```python
from build123d import *

# Parameters (mm, degrees)
F1_DEPTH = 31.75
F3_R     = 1.27
F4_R     = 4.7625
F4_R_2   = 4.1275
F5_DEPTH = 3.175
F6_R     = 4.7625
F6_R_2   = 4.1275
F7_DEPTH = 3.175


# Not quite as in the source:
# - a feature of the source that left no trace in its solid (it failed there, or was rolled back) is left out


with BuildPart() as f1:
    # F0 (on Right) → F1 (new body)
    with BuildSketch(Plane.YZ):
        Polygon((0, 203.2), (-304.8, 203.2), (-304.8, 200.025), (-228.6, 200.025), (-3.175, 76.2), (-3.175, 0), (0, 0), align=None)
        Polygon((-222.0052667175, 200.025), (-3.175, 200.025), (-3.175, 79.822459127), align=None, mode=Mode.SUBTRACT)
    extrude(amount=F1_DEPTH)

    # F3
    f3_edges = [f1.edges().sort_by_distance(p)[0] for p in [
        (15.875, -3.175, 79.822459),
        (15.875, -222.005267, 200.025),
        (15.875, -3.175, 200.025),
        (15.875, 0, 203.2),
        (15.875, -304.8, 203.2),
        (0, -152.4, 203.2),
        (31.75, -152.4, 203.2),
        (15.875, -304.8, 200.025),
        (0, -304.8, 201.6125),
        (31.75, -304.8, 201.6125),
        (0, -112.590133, 200.025),
        (31.75, -112.590133, 200.025),
        (15.875, 0, 0),
        (0, 0, 101.6),
        (31.75, 0, 101.6),
        (15.875, -3.175, 0),
        (0, -1.5875, 0),
        (31.75, -1.5875, 0),
        (15.875, -228.6, 200.025),
        (0, -266.7, 200.025),
        (31.75, -266.7, 200.025),
        (15.875, -3.175, 76.2),
        (0, -115.8875, 138.1125),
        (31.75, -115.8875, 138.1125),
        (0, -3.175, 38.1),
        (31.75, -3.175, 38.1),
        (0, -112.590133, 139.92373),
        (31.75, -112.590133, 139.92373),
        (0, -3.175, 139.92373),
        (31.75, -3.175, 139.92373),
    ]]
    fillet(f3_edges, radius=F3_R)

    # F4 (on face) → F5 (cut, through all)
    with BuildSketch(Plane(origin=(0, 0, 200.025), x_dir=(1, 0, 0), z_dir=(0, 0, -1))):
        with Locations((15.875, 285.75)):
            Circle(F4_R)
        with Locations((15.875, 247.65)):
            Circle(F4_R)
        with Locations((15.875, 146.05)):
            Circle(F4_R_2)
        with Locations((15.875, 44.45)):
            Circle(F4_R)
    extrude(amount=-F5_DEPTH, mode=Mode.SUBTRACT)

    # F6 (on face) → F7 (cut, through all)
    with BuildSketch(Plane.XZ.offset(3.175)):
        with Locations((15.875, 57.15)):
            Circle(F6_R)
        with Locations((15.875, 19.05)):
            Circle(F6_R)
        with Locations((15.875, 158.75)):
            Circle(F6_R_2)
    extrude(amount=-F7_DEPTH, mode=Mode.SUBTRACT)


solid = f1.part
```
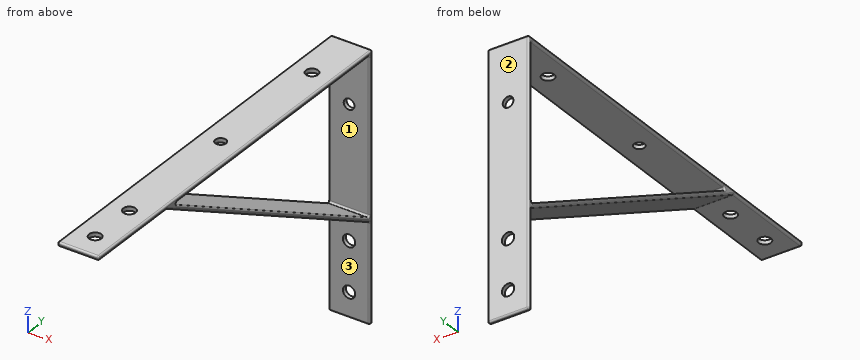
The model under review builds one solid part; all positions refer to its coordinate system, in mm. Face numbers are marked on the shaded views. A direction names the side the tool comes from. Give positions to 0.01 mm unless a question says otherwise; leave off trailing zeros. Write each loop counter-clockwise with the first axis right and the second up, starting at its lowest first coordinate (ties: lowest second). Pieces come first, ordered by that corner, then holes.
(1) Tool access review of the marked faces 1, 2 and 3: name each direction out of +Z, -Z, +X, -X, +Y, -Y from which nothing blocks a thin tool from reaching the whole face with its end or side.
(2) Consider section D-D, the plane z = 158.75. Give the number of separate pieces and of enclosed holes in the cut face, and give its area (3 significant figures).
(3) Consider section C-C, the plane z = 44. Give the boundary of the cut face in (x, y) (3 decimals), and give its area (3 significant figures).
(4) For P1, Ø5.5, axis at x = 15.875, y = -44.45, coming from the +Z side; P2, Ø4, axis at x = 12, y = -41, coming from the -Z side; P3, Ø6.5, axis at x = 15.875, z = 158.75, coming from the +Y side; P4, Ø5.5, axis at x = 15.875, z = 19.05, coming from the +Y side, all flat-tipped, find the tip position at first contact; note any pin that passes through.
(5) To check wall thickness, follow L1, parallel to X at y = -44.45, z = 201.35; L2, parallel to X at y = -44, z = 202; L3, parallel to Z at x = 22, y = -52.5 (3 decimals). State the ranges of each line that lie inside material, in increasing order.
Returned:
1. face 1: +X, -X
1. face 2: +Z, -Z, +X, -X, +Y
1. face 3: -Z, +X, -X, -Y
2. separate pieces: 3
2. enclosed holes: 0
2. area: 280 mm2
3. outline: (0, -1.905) arc R1.27 ccw to (1.27, -3.175) - (30.48, -3.175) arc R1.27 ccw to (31.75, -1.905) - (31.75, -1.27) arc R1.27 ccw to (30.48, 0) - (1.27, 0) arc R1.27 ccw to (0, -1.27) - close
3. area: 99.4 mm2
4. P1: stops at z = 104.01
4. P2: stops at z = 95.88
4. P3: stops at y = -140.95
4. P4: passes through
5. L1: x = 0 to 11.11, 20.64 to 31.75
5. L2: x = 0 to 11.13, 20.62 to 31.75
5. L3: z = 103.294 to 106.916, 200.025 to 203.2
